```python
from build123d import *

# Parameters (mm, degrees)
F1_DEPTH = 25.4
F2_R     = 6.35
F3_DEPTH = 25.4
F4_R     = 6.35
F5_DEPTH = 25.4
F6_R     = 6.35
F7_DEPTH = 25.4


with BuildPart() as f1:
    # F0 (on Front) → F1 (new body)
    with BuildSketch(Plane.XZ):
        Polygon((-16.770223, 14.04828), (-42.170223, 14.04828), (-42.170223, 1.34828), (34.029777, 1.34828), (34.029777, 14.04828), (8.629777, 14.04828), (8.629777, 39.44828), (-16.770223, 39.44828), align=None)
    extrude(amount=F1_DEPTH)

    # F2 (on face) → F3 (cut)
    with BuildSketch(Plane(origin=(-16.770223, 0, 0), x_dir=(0, -1, 0), z_dir=(-1, 0, 0))):
        with Locations((12.7, 26.74828)):
            Circle(F2_R)
        with BuildLine():
            ThreePointArc((0, 26.74828), (12.7, 38.797286), (25.4, 26.74828))
            Line((25.4, 26.74828), (25.4, 39.44828))
            Line((25.4, 39.44828), (0, 39.44828))
            Line((0, 39.44828), (0, 26.74828))
        make_face()
    extrude(amount=-F3_DEPTH, mode=Mode.SUBTRACT)

    # F4 (on face) → F5 (cut)
    with BuildSketch(Plane.XY.offset(14.04828)):
        with Locations((-29.470223, -12.7)):
            Circle(F4_R)
        with BuildLine():
            ThreePointArc((-29.470223, -25.4), (-41.771417, -12.7), (-29.470223, 0))
            Line((-29.470223, 0), (-42.170223, 0))
            Line((-42.170223, 0), (-42.170223, -25.4))
            Line((-42.170223, -25.4), (-29.470223, -25.4))
        make_face()
    extrude(amount=-F5_DEPTH, mode=Mode.SUBTRACT)

    # F6 (on face) → F7 (cut)
    with BuildSketch(Plane.XY.offset(14.04828)):
        with Locations((21.329777, -12.7)):
            Circle(F6_R)
        with BuildLine():
            ThreePointArc((21.329777, 0), (33.774057, -12.7), (21.329777, -25.4))
            Line((21.329777, -25.4), (34.029777, -25.4))
            Line((34.029777, -25.4), (34.029777, 0))
            Line((34.029777, 0), (21.329777, 0))
        make_face()
    extrude(amount=-F7_DEPTH, mode=Mode.SUBTRACT)


solid = f1.part
```
Read the model definition and answer for the solid it produces. Units are mm, in the model's axes. A direction names the side the tool comes from. Round coordinates to 2 decimals unless told otherwise and drop trailing zeros. Write each loop counter-clockwise with the first axis right and the second up, starting at its lowest first coordinate (ties: lowest second). Pieces come first, ordered by that corner, then holes. Notation, with made-up numbers: (39.25, -31) - (77.25, -31) arc R29 ccw to (77.25, 1) - close; hole circle Ø3 at (31, 76). An arc over 180 degrees is marked (long way). One line per item, written item: value.
Q1. Straight lines are drawn through the part: line 1 (X direction, y = -13, z = 8.5); line 2 (Z direction, x = 6, y = -13); line 3 (X direction, y = -8, z = 10). For each, find the intervals that lie inside material, in ascending order. Write a range as from..to.
The answers:
line 1: x = -41.77..-35.81, -23.13..14.99, 27.67..33.77
line 2: z = 1.35..20.41, 33.09..38.79
line 3: x = -40.87..-33.74, -25.2..17.06, 25.6..32.87
Q2. Find section A-A (y = -12.7). Determine the outline of the cut face in (x, z), and give its area (3 significant figures).
The answers:
outline: (-41.77, 1.35) - (-35.82, 1.35) - (-35.82, 14.05) - (-41.77, 14.05) - close; (-23.12, 1.35) - (14.98, 1.35) - (14.98, 14.05) - (8.63, 14.05) - (8.63, 20.4) - (-16.77, 20.4) - (-16.77, 14.05) - (-23.12, 14.05) - close; (-16.77, 33.1) - (8.63, 33.1) - (8.63, 38.8) - (-16.77, 38.8) - close; (27.68, 1.35) - (33.77, 1.35) - (33.77, 14.05) - (27.68, 14.05) - close
area: 943 mm2
Q3. For a pull along Y with two mould halves and no side action, classify faces 1 (the flat face through (-4, -25.4, 11)), 2 (the cylindrical face through (-4.248, -12.43, 38.794)), 3 (the flat face through (8.63, -15.3, 20.7)), 4 (the cylindrical face through (-4.25, -11.32, 20.55)) as pulls with the +Y half, pulls with the -Y half, needs draft (parallel to the pull), parting line crosses it, or undercut.
The answers:
face 1: pulls with the -Y half
face 2: parting line crosses it
face 3: needs draft
face 4: undercut
Q4. Which of the six approach directions +Z, -Z, +X, -X, +Y, -Y give full straight-line access (tool end or side, diameter ignored) to faces 5 (the flat face through (-16.77, -6.9, 23.8)), 6 (the flat face through (-5, -13, 1.348)), 7 (the flat face through (13, -13, 14.048))?
The answers:
face 5: +Z, -X, +Y, -Y
face 6: -Z, +X, -X, +Y, -Y
face 7: +Z, +X, +Y, -Y
Q5. Each of these flat-tipped pins is pushed along its axis until it touches: P1, Ø12.5, axis at x = -32.5, y = -9.5, coming from the +Z side; P2, Ø1, axis at y = -11.5, z = 21.5, coming from the -X side; P3, Ø12.5, axis at y = -8, z = 28.5, coming from the +X side; P4, Ø4, axis at x = -12.5, y = -20.5, coming from the +Z side. Where does it stop, or does it pass through?
The answers:
P1: stops at z = 14.05
P2: passes through
P3: stops at x = 8.63
P4: stops at z = 37.4
Q6. Find section C-C (z = 23.5). Determine the outline of the cut face in (x, y), and give its area (3 significant figures).
The answers:
outline: (-16.77, -25.4) - (8.63, -25.4) - (8.63, -18.16) - (-16.77, -18.16) - close; (-16.77, -7.24) - (8.63, -7.24) - (8.63, 0) - (-16.77, 0) - close
area: 368 mm2
Q7. Find section B-B (x = 7). Determine the outline of the cut face in (y, z), and give its area (3 significant figures).
The answers:
outline: (-25.4, 1.35) - (0, 1.35) - (0, 26.75) arc R12.72 ccw to (-25.4, 26.75) - close; hole circle Ø12.7 at (-12.7, 26.75)
area: 756 mm2
Q8. Find section D-D (z = 5). Determine the outline of the cut face in (x, y).
The answers:
outline: (-29.47, -25.4) - (21.33, -25.4) arc R12.7 ccw to (21.33, 0) - (-29.47, 0) arc R12.71 ccw to start; hole circle Ø12.7 at (-29.47, -12.7); hole circle Ø12.7 at (21.33, -12.7)
